Read the model definition and answer for the solid it produces. Units are mm, in the model's axes. A direction names the side the tool comes from. Give positions to 0.01 mm unless a question says otherwise; leave off trailing zeros. Order: outer loops, then holes, each group sorted by start corner. A loop starts at its lowest first (then second) coordinate and runs counter-clockwise, first axis right, second up. Notation, with made-up numbers: (0, 48.25) -> (25, 48.25) arc R23 ccw to (25, 60.25) -> close; hole circle Ø1 at (-26, -6). An arc over 180 degrees is marked (long way). Use one line per item in the form item = value.
```python
from build123d import *

# Parameters (mm, degrees)
SKETCH1_W           = 50.8
SKETCH1_H           = 20.32
SKETCH1_R           = 1.4732
BOSS_EXTRUDE1_DEPTH = 4.826
SKETCH2_W           = 50.8
SKETCH2_H           = 4.826
BOSS_EXTRUDE2_DEPTH = 26.924
FILLET1_R           = 2.54
SKETCH3_R           = 4.8133
CUT_EXTRUDE1_DEPTH  = 26.924


with BuildPart() as part:
    # Sketch1 → Boss-Extrude1 (new body)
    with BuildSketch(Plane(origin=(0, 0, 0), x_dir=(1, 0, 0), z_dir=(0, 1, 0))):
        with Locations((25.4, 10.16)):
            Rectangle(SKETCH1_W, SKETCH1_H)
        with Locations(Location((12.7, 10.16, 0), (0, 0, 270))):
            Circle(SKETCH1_R, mode=Mode.SUBTRACT)
        with Locations(Location((38.1, 10.16, 0), (0, 0, 270))):
            Circle(SKETCH1_R, mode=Mode.SUBTRACT)
    extrude(amount=BOSS_EXTRUDE1_DEPTH)

    # Sketch2 → Boss-Extrude2 (add)
    with BuildSketch(Plane(origin=(0, 4.826, 0), x_dir=(1, 0, 0), z_dir=(0, 1, 0))):
        with Locations((25.4, 17.907)):
            Rectangle(SKETCH2_W, SKETCH2_H)
    extrude(amount=BOSS_EXTRUDE2_DEPTH)

    # Fillet1
    fillet1_edges = [part.edges().sort_by_distance(p)[0] for p in [
        (25.4, 31.75, -15.494),
        (25.4, 4.826, 0),
    ]]
    fillet(fillet1_edges, radius=FILLET1_R)

    # Sketch3 → Cut-Extrude1 (cut)
    with BuildSketch(Plane(origin=(0, 0, -20.32), x_dir=(-1, 0, 0), z_dir=(0, 0, -1))):
        with Locations((-38.1, 19.05)):
            Circle(SKETCH3_R)
        with Locations((-12.7, 19.05)):
            Circle(SKETCH3_R)
    extrude(amount=-CUT_EXTRUDE1_DEPTH, mode=Mode.SUBTRACT)


solid = part.part
```
Item 1: The part is cut by section C-C on x = 12.7. Give the vertices of the cut face in (y, z).
Checks:
outline = (0, -20.32) -> (14.24, -20.32) -> (14.24, -15.49) -> (4.83, -15.49) -> (4.83, -11.63) -> (0, -11.63) -> close; (0, -8.69) -> (4.83, -8.69) -> (4.83, -2.54) arc R2.54 ccw to (2.29, 0) -> (0, 0) -> close; (23.86, -20.32) -> (31.75, -20.32) -> (31.75, -18.03) arc R2.54 ccw to (29.21, -15.49) -> (23.86, -15.49) -> close
Item 2: Straight lines are drawn through the part: L1, parallel to X at y = 2.2, z = -10.16; L2, parallel to Y at x = 12.7, z = -18.35. For each, find the intervals that lie inside material, in ascending order. Write a range as from..to.
Checks:
L1 = 0..11.23, 14.17..36.63, 39.57..50.8
L2 = 0..14.24, 23.86..31.75
Item 3: Which of the six approach directions +Z, -Z, +X, -X, +Y, -Y give full straight-line access (tool end or side, diameter ignored) to faces 5 (the cylindrical face through (36.66, 2.38, -10.48)), 6 (the flat face through (25, 4.826, -9))?
Checks:
face_5 = +Y, -Y
face_6 = +Z, +X, -X, +Y
Item 4: Determine the mould class of faces 1 (the flat face through (50.8, 12, -16)), 2 (the flat face through (25, 31.75, -19)), 3 (the flat face through (25, 0, -10)), 4 (the cylindrical face through (33.654, 17.206, -17.941)) for opening direction Y: +Y half, -Y half, draft (parallel to the pull), parting line (faces both ways), or undercut.
Checks:
face_1 = draft
face_2 = +Y half
face_3 = -Y half
face_4 = undercut
Item 5: Given pin 1 Ø2.5 at (x, z) = (38.1, -10.16) entering from +Y; pin 2 Ø7.5 at (x, y) = (20, 14.5) entering from +Z; pin 3 Ø6.5 at (x, z) = (27.5, -9) entering from +Y, each flat-ended and moving along its own axis, determine where each tip first touches the part or whether it passes through.
Checks:
pin_1 = through
pin_2 = -15.49
pin_3 = 4.83
Item 6: The part is cut by section D-D on x = 46.5. Give the vertices of the cut face in (y, z).
Checks:
outline = (0, -20.32) -> (31.75, -20.32) -> (31.75, -18.03) arc R2.54 ccw to (29.21, -15.49) -> (4.83, -15.49) -> (4.83, -2.54) arc R2.54 ccw to (2.29, 0) -> (0, 0) -> close
Item 7: The part is cut by section A-A on y = 19.05. Give the vertices of the cut face in (x, z).
Checks:
outline = (0, -20.32) -> (7.89, -20.32) -> (7.89, -15.49) -> (0, -15.49) -> close; (17.51, -20.32) -> (33.29, -20.32) -> (33.29, -15.49) -> (17.51, -15.49) -> close; (42.91, -20.32) -> (50.8, -20.32) -> (50.8, -15.49) -> (42.91, -15.49) -> close
Item 8: The part is cut by section B-B on z = -10.16. Give the vertices of the cut face in (x, y), and give its area (3 significant figures).
Checks:
outline = (0, 0) -> (11.23, 0) -> (11.23, 4.83) -> (0, 4.83) -> close; (14.17, 0) -> (36.63, 0) -> (36.63, 4.83) -> (14.17, 4.83) -> close; (39.57, 0) -> (50.8, 0) -> (50.8, 4.83) -> (39.57, 4.83) -> close
area = 217 mm²
